Geometry: final body of the model. Coordinates: model frame, mm. A direction names the side the tool comes from. Give positions to 0.01 mm unless a question says otherwise; leave off trailing zeros. Write each loop counter-clockwise with the first axis right and the second up, starting at its lowest first coordinate (ties: lowest second). Pieces come first, ordered by that corner, then holes.
```python
from build123d import *

# Parameters (mm, degrees)
SKETCH1_R                = 3
BOSS_EXTRUDE2_DEPTH      = 6
M4_CLEARANCE_HOLE1_D     = 4.5
M4_CLEARANCE_HOLE1_DEPTH = 84
M4_CLEARANCE_HOLE1_TIP   = 1.351936393
CUT_EXTRUDE1_DEPTH       = 203.576880123
M3_CLEARANCE_HOLE1_D     = 3.4


with BuildPart() as part:
    # Sketch1 → Boss-Extrude2 (new body)
    with BuildSketch(Plane.XY):
        with BuildLine():
            Line((139.718429351, 20.947970782), (171.818869964, 33.969557183))
            ThreePointArc((171.818869964, 33.969557183), (197.870084408, 22.954375569), (186.854902793, -3.096838875))
            Line((186.854902793, -3.096838875), (144.82255129, -20.147318131))
            Line((144.82255129, -20.147318131), (39.618457028, -5.511611627))
            Line((39.618457028, -5.511611627), (7.518016414, -18.533198029))
            ThreePointArc((7.518016414, -18.533198029), (-18.533198029, -7.518016414), (-7.518016414, 18.533198029))
            Line((-7.518016414, 18.533198029), (34.514335089, 35.583677285))
            Line((34.514335089, 35.583677285), (139.718429351, 20.947970782))
        make_face()
        with Locations((179.336886379, 15.436359154)):
            Circle(SKETCH1_R, mode=Mode.SUBTRACT)
        Circle(SKETCH1_R, mode=Mode.SUBTRACT)
    extrude(amount=BOSS_EXTRUDE2_DEPTH)

    # M4 Clearance Hole1
    with Locations(Plane(origin=(35.535159477, 27.364619503, 6), x_dir=(1, 0, 0), z_dir=(0, 0, 1))):
        with Locations((0, 0), (108.266567425, -39.292879851), (3.118996753, -25.112266952), (105.147570672, -14.1806129), (54.133283712, -19.646439926)):
            Hole(M4_CLEARANCE_HOLE1_D / 2, depth=M4_CLEARANCE_HOLE1_DEPTH)
            with Locations((0, 0, -(M4_CLEARANCE_HOLE1_DEPTH + M4_CLEARANCE_HOLE1_TIP / 2))):  # 118° drill point
                Cone(0, M4_CLEARANCE_HOLE1_D / 2, M4_CLEARANCE_HOLE1_TIP, mode=Mode.SUBTRACT)

    # Sketch5 → Cut-Extrude1 (cut, through all)
    with BuildSketch(Plane.XY.offset(6)):
        with BuildLine():
            Line((128.460158473, -3.736200604), (103.698622831, -0.291443337))
            ThreePointArc((103.698622831, -0.291443337), (98.582596021, 6.478066961), (105.352106319, 11.594093771))
            Line((105.352106319, 11.594093771), (130.113641961, 8.149336504))
            ThreePointArc((130.113641961, 8.149336504), (135.229668771, 1.379826206), (128.460158473, -3.736200604))
        make_face()
        with BuildLine():
            Line((73.98478006, 3.842265383), (49.223244417, 7.28702265))
            ThreePointArc((49.223244417, 7.28702265), (44.107217607, 14.056532949), (50.876727906, 19.172559759))
            Line((50.876727906, 19.172559759), (75.638263548, 15.727802492))
            ThreePointArc((75.638263548, 15.727802492), (80.754290358, 8.958292193), (73.98478006, 3.842265383))
        make_face()
    extrude(amount=-CUT_EXTRUDE1_DEPTH, mode=Mode.SUBTRACT)

    # M3 Clearance Hole1 (through all)
    with Locations(Plane(origin=(182.43806815, 7.791414967, 6), x_dir=(1, 0, 0), z_dir=(0, 0, 1))):
        with Locations((0, 0), (-6.202363542, 15.289888374), (-185.539249921, -0.14647078), (-179.336886379, -15.436359154)):
            Hole(M3_CLEARANCE_HOLE1_D / 2)


solid = part.part
```
Item 1: Pin query (flat end, axial travel): pin 1 Ø3 at (x, z) = (80.5, 1) entering from +Y; pin 2 Ø1 at (y, z) = (1.5, 4.5) entering from +X; pin 3 Ø3 at (y, z) = (-12.5, 4) entering from -X. Return the tip coordinate at first contact, or that it passes through.
Found:
pin 1: stops at y = 29.39
pin 2: stops at x = 194.15
pin 3: stops at x = -16.7
Item 2: Line query: L1, parallel to Y at x = -2.5, z = 4.25; L2, parallel to Y at x = 0, z = 2; L3, parallel to Y at x = 80, z = 3.5. Output: solid intervals per line, ascending.
Found:
L1: y = -19.84 to -1.66, 1.66 to 6.05, 9.24 to 20.57
L2: y = -20 to -3, 3 to 21.58
L3: y = -11.13 to 6.77, 12.8 to 29.26
Item 3: Section A-A, the plane x = 11.5. Return the cut outline in (y, z), plus the area to 3 significant figures.
Found:
outline: (-16.92, 0) - (26.25, 0) - (26.25, 6) - (-16.92, 6) - close
area: 259 mm2
Item 4: Pull-direction query (Y, two-part tool) for faces 1 (the face through (36.576, 1.391, 2.958)), 2 (the face through (13.204, 26.939, 2.958)), 3 (the face through (183.79, 6.76, 2.96)), 4 (the face through (91, 2, 0)); classes: +Y half, -Y half, draft (parallel to the pull), parting line (faces both ways), or undercut.
Found:
face 1: undercut
face 2: +Y half
face 3: undercut
face 4: draft
Item 5: Reachability of faces 5 (the face through (86.38, 28.37, 2.96)), 6 (the face through (44.09, 13.93, 3.04)), 7 (the face through (92.957, -12.932, 2.958)) from +Z, -Z, +X, -X, +Y, -Y: full face, straight path, thin tool, end or side. Return the list, or none.
Found:
face 5: +Z, -Z, +Y
face 6: +Z, -Z
face 7: +Z, -Z, -Y
